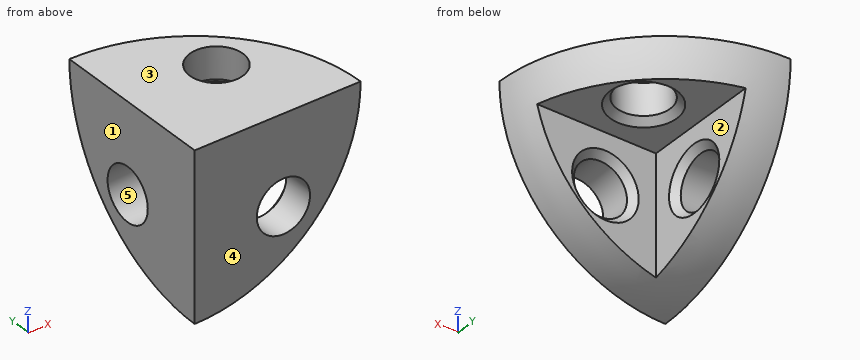
```python
from build123d import *

# Parameters (mm, degrees)
REVOLVE_1_ANGLE     = 90
SHELL_3_T           = -4.3
SKETCH_1_3_R        = 3
CUT_EXTRUDE_2_DEPTH = 10
SKETCH_3_R          = 3
CUT_EXTRUDE_3_DEPTH = 10
SKETCH_4_R          = 3
CUT_EXTRUDE_4_DEPTH = 10
CHAMFER_1_SIZE      = 0.75


with BuildPart() as part:
    # Sketch 1 → Revolve 1 (revolve)
    with BuildSketch(Plane.XY):
        with BuildLine():
            Line((0, 0), (18.7, 0))
            ThreePointArc((18.7, 0), (13.222896808, 13.222896808), (0, 18.7))
            Line((0, 18.7), (0, 0))
        make_face()
    revolve(axis=Axis((0, 0, 0), (0, 1, 0)), revolution_arc=REVOLVE_1_ANGLE)

    # Shell 3
    shell_3_openings = [part.faces().sort_by_distance(p)[0] for p in [
        (9.35, 13.222896808, -9.35),
    ]]
    offset(amount=SHELL_3_T, openings=shell_3_openings, kind=Kind.INTERSECTION)

    # Sketch 1_3 → Cut-Extrude 2 (cut)
    with BuildSketch(Plane.XY):
        with Locations((10, 10)):
            Circle(SKETCH_1_3_R)
    extrude(amount=-CUT_EXTRUDE_2_DEPTH, mode=Mode.SUBTRACT)

    # Sketch 3 → Cut-Extrude 3 (cut)
    with BuildSketch(Plane.XZ):
        with Locations(Location((10, -10, 0), (0, 0, 270))):
            Circle(SKETCH_3_R)
    extrude(amount=-CUT_EXTRUDE_3_DEPTH, mode=Mode.SUBTRACT)

    # Sketch 4 → Cut-Extrude 4 (cut)
    with BuildSketch(Plane.ZY):
        with Locations((-10, 10)):
            Circle(SKETCH_4_R)
    extrude(amount=-CUT_EXTRUDE_4_DEPTH, mode=Mode.SUBTRACT)

    # Chamfer 1
    chamfer_1_edges = [part.edges().sort_by_distance(p)[0] for p in [
        (7, 10, -4.3),
        (10, 4.3, -7),
        (4.3, 10, -13),
    ]]
    chamfer(chamfer_1_edges, length=CHAMFER_1_SIZE)


solid = part.part
```
Check sheet for the modelled part. Datum: model origin and axes. Units: mm. Face numbers are marked on the shaded views. A direction names the side the tool comes from. Coordinates: 2 decimals unless noted, no trailing zeros. Write each loop counter-clockwise with the first axis right and the second up, starting at its lowest first coordinate (ties: lowest second). Pieces come first, ordered by that corner, then holes. Notation, with made-up numbers: M 34.5,73.5 L 88.5,73.5 A19 ccw 88.5,98.5 Z; hole C 69,46 d9. An arc over 180 degrees is marked long. Use one line per item in the form item = value.
Item 1: Gauge pin test, flat ends, axial feed: pin 1 Ø3 at (x, z) = (9.5, -14) entering from +Y; pin 2 Ø4 at (y, z) = (8, -14) entering from +X; pin 3 Ø4 at (x, y) = (10.5, 6) entering from -Z. Record the tip position at first contact, or that the pin passes through.
Answer below:
pin_1 = 4.3
pin_2 = 4.3
pin_3 = -15.56
Item 2: Sectioned sample at A-A, the plane y = 10. Record the cut outline in (x, z), and give its area (3 significant figures).
Answer below:
outline = M 0,-15.8 A15.8 ccw 4.3,-15.21 L 4.3,-13.75 L 3.55,-13 L 0,-13 Z; M 0,-7 L 3.55,-7 L 4.3,-6.25 L 4.3,-4.3 L 6.25,-4.3 L 7,-3.55 L 7,0 L 0,0 Z; M 13,-3.55 L 13.75,-4.3 L 15.21,-4.3 A15.8 ccw 15.8,0 L 13,0 Z
area = 63.0 mm^2
Item 3: Release check for a two-part mould opening along Z. For the marked faces 3, 4 and 5 record: pulls with the +Z half, pulls with the -Z half, needs draft (parallel to the pull), parting line crosses it, or undercut.
Answer below:
face_3 = pulls with the +Z half
face_4 = needs draft
face_5 = undercut
Item 4: Material ranges on L1, parallel to Z at x = 4, y = 7.25; L2, parallel to Y at x = 1.5, z = -7.75; L3, parallel to X at y = 2, z = -10, recorded low to high. Write a range as from..to.
Answer below:
L1 = -16.77..-12.08, -7.92..0
L2 = 0..8.02, 11.98..16.95
L3 = 0..7, 13..15.67
Item 5: Sectioned sample at C-C, the plane x = 16.5. Record the cut outline in (y, z).
Answer below:
outline = M 0,-8.8 A8.8 ccw 4.3,-7.68 L 4.3,-4.3 L 7.68,-4.3 A8.8 ccw 8.8,0 L 0,0 Z
Item 6: Set-up check for the marked faces 1 and 2: record each of +Z, -Z, +X, -X, +Y, -Y from which the full face is reachable in a straight line by a thin tool's end or side.
Answer below:
face_1 = +Z, -Z, -X, +Y, -Y
face_2 = -Z, +X, +Y
Item 7: Sectioned sample at B-B, the plane z = -8.5. State how many separate pieces and enclosed holes the cut face has, and give its area (3 significant figures).
Answer below:
separate_pieces = 3
enclosed_holes = 0
area = 77.2 mm^2
